Here's how the part is built. I have some questions about the finished solid (model axes, mm). Face numbers are marked on the shaded views. Coordinates: 2 decimals unless noted, no trailing zeros. Write each loop counter-clockwise with the first axis right and the second up, starting at its lowest first coordinate (ties: lowest second). Pieces come first, ordered by that corner, then holes. Notation, with made-up numbers: (-29, 9) - (-16, 9) arc R20 cw to (-16, 24) - close; hole circle Ø10 at (81.25, -11.5). An arc over 180 degrees is marked (long way). Answer in a Markdown table with one row per item. Add a question column.
Item 1: Imagine slicing it at C-C (x = 57). Please give me the cut outline in (y, z).
Item 2: Imagine slicing it at B-B (z = -57). Please give me the cut outline in (x, y), plus the area to 3 significant figures.
Item 3: We'd pull the mould along Y, two halves only. Please class the marked faces 1 and 2: +Y half, -Y half, draft (parallel to the pull), parting line (faces both ways), or undercut.
Item 4: If I drill on probe 1 along Z at (x, y) = (-57, 5); probe 2 along X at (y, z) = (6.25, 0); probe 3 along Z at (x, y) = (-60, 7.5), over which ranges is the centre line in solid material (lowest first)? Write a range as from..to.
Item 5: I'm going to push a flat-ended pin straight in: pin 1 (10.5 mm diameter, centred on x = -57, z = 57, fed in from +Y). Where does the tip first touch, or does it pass through?
Item 6: Imagine slicing it at A-A (x = -50). Please give me the cut outline in (y, z), plus the area to 3 significant figures.
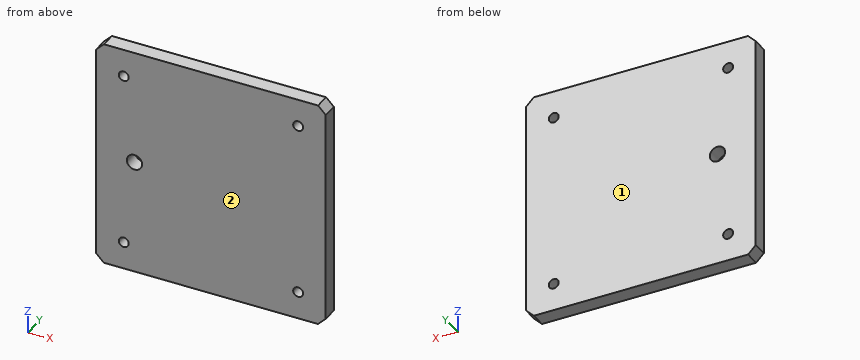
from build123d import *

# Parameters (mm, degrees)
SKETCH1_W            = 150
SKETCH1_H            = 150
BOSS_EXTRUDE1_DEPTH  = 10
CHAMFER1_SIZE        = 5
M6_CLEARANCE_HOLE1_D = 6.5
SKETCH2_R            = 5
CUT_EXTRUDE1_DEPTH   = 15


with BuildPart() as part:
    # Sketch1 → Boss-Extrude1 (new body)
    with BuildSketch(Plane(origin=(0, 0, 0), x_dir=(1, 0, 0), z_dir=(0, 1, 0))):
        Rectangle(SKETCH1_W, SKETCH1_H)
    extrude(amount=BOSS_EXTRUDE1_DEPTH)

    # Chamfer1
    chamfer1_edges = [part.edges().sort_by_distance(p)[0] for p in [
        (-75, 5, -75),
        (75, 5, -75),
        (75, 5, 75),
        (-75, 5, 75),
    ]]
    chamfer(chamfer1_edges, length=CHAMFER1_SIZE)

    # M6 Clearance Hole1 (through all)
    with Locations(Plane(origin=(0, 10, 0), x_dir=(-1, 0, 0), z_dir=(0, 1, 0))):
        with Locations((57, -57), (-57, -57), (57, 57), (-57, 57)):
            Hole(M6_CLEARANCE_HOLE1_D / 2)

    # Sketch2 → Cut-Extrude1 (cut)
    with BuildSketch(Plane(origin=(0, 10, 0), x_dir=(1, 0, 0), z_dir=(0, 1, 0))):
        with Locations(Location((-50, 0, 0), (0, 0, 270))):
            Circle(SKETCH2_R)
    extrude(amount=-CUT_EXTRUDE1_DEPTH, mode=Mode.SUBTRACT)


solid = part.part
Here are the results:
| question | item | result |
|---|---|---|
| 1 | outline | (0, -75) - (10, -75) - (10, -60.25) - (0, -60.25) - close; (0, -53.75) - (10, -53.75) - (10, 53.75) - (0, 53.75) - close; (0, 60.25) - (10, 60.25) - (10, 75) - (0, 75) - close |
| 2 | outline | (-75, 0) - (-60.25, 0) - (-60.25, 10) - (-75, 10) - close; (-53.75, 0) - (53.75, 0) - (53.75, 10) - (-53.75, 10) - close; (60.25, 0) - (75, 0) - (75, 10) - (60.25, 10) - close |
| 2 | area | 1,370 mm2 |
| 3 | face 1 | +Y half |
| 3 | face 2 | -Y half |
| 4 | probe 1 | z = -75..-60.25, -53.75..53.75, 60.25..75 |
| 4 | probe 2 | x = -75..-55, -45..75 |
| 4 | probe 3 | z = -75..-58.25, -55.75..55.75, 58.25..75 |
| 5 | pin 1 | stops at y = 10 |
| 6 | outline | (0, -75) - (10, -75) - (10, -5) - (0, -5) - close; (0, 5) - (10, 5) - (10, 75) - (0, 75) - close |
| 6 | area | 1,400 mm2 |
